Input: part model. Units: mm. Frame: model coordinates. Face numbers are marked on the shaded views. A direction names the side the tool comes from. Coordinates: 2 decimals unless noted, no trailing zeros. Write each loop counter-clockwise with the first axis right and the second up, starting at its lowest first coordinate (ties: lowest second). Pieces come first, ordered by that corner, then holes. Notation, with made-up numbers: (77.5, 45.5) - (94.5, 45.5) arc R28 ccw to (94.5, 81.5) - close; hole circle Ø2 at (61, 30). An arc over 180 degrees is marked (long way). Use a Markdown table: item, result. Add a question column.
Q1. Section query A-A (z = 35). Return the cut outline in (x, y).
Q2. Pin query (flat end, axial travel): P1, Ø1.5, axis at x = -2, y = -1, coming from the -Z side; P2, Ø1.6, axis at y = 1.5, z = -39.5, coming from the -X side; P3, Ø3, axis at y = -3.5, z = -8, coming from the -X side. Return the tip coordinate at first contact, or that it passes through.
Q3. Section query B-B (x = 14). Return the cut outline in (y, z).
Q4. Material intervals for probe 1 along X at (y, z) = (2.1, 0); probe 2 along Z at (x, y) = (-23, 0.8); probe 3 along Z at (x, y) = (-24, 1.5), sorted ascending. Write a range as from..to.
Q5. Section query C-C (z = 18.5). Return the cut outline in (x, y), then the cut area to 3 significant figures.
Q6. Set-up query: the marked faces 1, 2 and 3. Return all of +Z, -Z, +X, -X, +Y, -Y with unobstructed straight access to the full face (end or side cutting, diameter ignored); none if empty.
Q7. Section query D-D (z = -5.5). Return the cut outline in (x, y), then the cut area to 3 significant figures.
from build123d import *

# Parameters (mm, degrees)
A_BASE_T42_OUTLINE_R              = 2.2479
A_BASE_T42_OUTLINE_R_2            = 1
A_BASE_T42_DEPTH                  = 3
OUTER_RIM_CUT_DEPTH               = 68.299702823
SKETCH2_W                         = 20
SKETCH2_H                         = 3
FLANGES_DEPTH                     = 3
CONTOURING_R                      = 1
SKETCH3_W                         = 15
SKETCH3_H                         = 3
BASE_SUPPORTS_DEPTH               = 3
BASE_SUPPORTS_CHAMFER_SIZE        = 3
SKETCH4_W                         = 3
SKETCH4_H                         = 45
DYNAMIXEL_SIDE_SUPPORTS_DEPTH     = 6.85
SKETCH5_W                         = 12
SKETCH5_H                         = 3
DYNAMIXEL_SIDE_SUPPORT_ENDS_DEPTH = 9.85
SKETCH8_W                         = 9
SKETCH8_H                         = 45
DYNAMIXEL_OFFSET_DEPTH            = 1.25
DYNAMIXEL_CONTOURING_R            = 1


# Read off the part's stored shape, not the designer's step: a_base_t42
with BuildPart() as part:
    # a_base_t42 outline → a_base_t42 (new body)
    with BuildSketch(Plane(origin=(0, 0, 0), x_dir=(1, 0, 0), z_dir=(0, 1, 0))):
        with BuildLine():
            ThreePointArc((31.5, -42), (52.5, 0), (31.5, 42))
            Line((31.5, 42), (-31.5, 42))
            ThreePointArc((-31.5, 42), (-52.5, 0), (-31.5, -42))
            Line((-31.5, -42), (31.5, -42))
        make_face()
        with Locations((-23, -35)):
            Circle(A_BASE_T42_OUTLINE_R, mode=Mode.SUBTRACT)
        with Locations((23, -35)):
            Circle(A_BASE_T42_OUTLINE_R, mode=Mode.SUBTRACT)
        with Locations((-40.25, 0)):
            Circle(A_BASE_T42_OUTLINE_R_2, mode=Mode.SUBTRACT)
        with Locations((-23, 35)):
            Circle(A_BASE_T42_OUTLINE_R, mode=Mode.SUBTRACT)
        with Locations((40.25, 0)):
            Circle(A_BASE_T42_OUTLINE_R_2, mode=Mode.SUBTRACT)
        with Locations((23, 35)):
            Circle(A_BASE_T42_OUTLINE_R, mode=Mode.SUBTRACT)
    extrude(amount=A_BASE_T42_DEPTH)

    # Sketch1 → Outer Rim Cut (cut, through all)
    with BuildSketch(Plane.XZ):
        with BuildLine():
            Line((31.5, 42), (-31.5, 42))
            ThreePointArc((-31.5, 42), (-52.5, 0), (-31.5, -42))
            Line((-31.5, -42), (31.5, -42))
            ThreePointArc((31.5, -42), (52.5, 0), (31.5, 42))
        make_face()
        with BuildLine():
            Line((30.483602149, 39), (-30.483602149, 39))
            ThreePointArc((-30.483602149, 39), (-49.5, 0), (-30.483602149, -39))
            Line((-30.483602149, -39), (30.483602149, -39))
            ThreePointArc((30.483602149, -39), (49.5, 0), (30.483602149, 39))
        make_face(mode=Mode.SUBTRACT)
    extrude(amount=-OUTER_RIM_CUT_DEPTH, mode=Mode.SUBTRACT)

    # Sketch2 → Flanges (add)
    with BuildSketch(Plane.XZ):
        with Locations((0, -40.5)):
            Rectangle(SKETCH2_W, SKETCH2_H)
        with Locations((0, 40.5)):
            Rectangle(SKETCH2_W, SKETCH2_H)
    extrude(amount=-FLANGES_DEPTH)

    # Contouring
    contouring_edges = [part.edges().sort_by_distance(p)[0] for p in [
        (30.483602149, 1.5, -39),
        (-30.483602149, 1.5, -39),
        (10, 1.5, -42),
        (-10, 1.5, -42),
        (30.483602149, 1.5, 39),
        (-30.483602149, 1.5, 39),
        (10, 1.5, 42),
        (-10, 1.5, 42),
    ]]
    fillet(contouring_edges, radius=CONTOURING_R)

    # Sketch3 → Base Supports (add)
    with BuildSketch(Plane.XZ):
        with Locations((0, -27)):
            Rectangle(SKETCH3_W, SKETCH3_H)
        with Locations((0, 27)):
            Rectangle(SKETCH3_W, SKETCH3_H)
    extrude(amount=BASE_SUPPORTS_DEPTH)

    # Base Supports Chamfer
    base_supports_chamfer_edges = [part.edges().sort_by_distance(p)[0] for p in [
        (0, 0, 28.5),
        (0, 0, -28.5),
    ]]
    chamfer(base_supports_chamfer_edges, length=BASE_SUPPORTS_CHAMFER_SIZE - 0.0001)  # a hair under: the kernel refuses the full size

    # Sketch4 → Dynamixel Side Supports (add)
    with BuildSketch(Plane.XZ):
        with Locations((-32.5, 0)):
            Rectangle(SKETCH4_W, SKETCH4_H)
        with Locations((32.5, 0)):
            Rectangle(SKETCH4_W, SKETCH4_H)
    extrude(amount=DYNAMIXEL_SIDE_SUPPORTS_DEPTH)

    # Sketch5 → Dynamixel Side Support Ends (add)
    with BuildSketch(Plane.XZ):
        with Locations((-28, 24)):
            Rectangle(SKETCH5_W, SKETCH5_H)
        with Locations((28, -24)):
            Rectangle(SKETCH5_W, SKETCH5_H)
    extrude(amount=DYNAMIXEL_SIDE_SUPPORT_ENDS_DEPTH)

    # Sketch8 → Dynamixel Offset (add)
    with BuildSketch(Plane.XZ):
        with Locations((-26.5, 0)):
            Rectangle(SKETCH8_W, SKETCH8_H)
        with Locations((26.5, 0)):
            Rectangle(SKETCH8_W, SKETCH8_H)
    extrude(amount=DYNAMIXEL_OFFSET_DEPTH)

    # Dynamixel Contouring
    dynamixel_contouring_edges = [part.edges().sort_by_distance(p)[0] for p in [
        (-31, -4.05, -22.5),
        (31, -4.05, 22.5),
        (-34, -4.925, 25.5),
        (-22, -5.55, 22.5),
        (-28, -9.85, 22.5),
        (34, -4.925, -25.5),
        (22, -5.55, -22.5),
        (28, -9.85, -22.5),
        (-22, -0.625, -22.5),
        (22, -0.625, 22.5),
    ]]
    fillet(dynamixel_contouring_edges, radius=DYNAMIXEL_CONTOURING_R)


solid = part.part
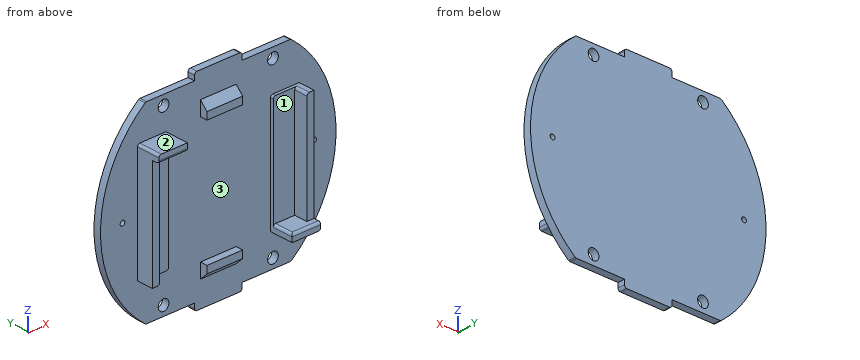
Values follow:
| question | item | result |
|---|---|---|
| 1 | outline | (-35, 0) - (-25.25, 0) - (-25.25, 3) - (-35, 3) - close; (-20.75, 0) - (20.75, 0) - (20.75, 3) - (-20.75, 3) - close; (25.25, 0) - (35, 0) - (35, 3) - (25.25, 3) - close |
| 2 | P1 | z = -31.25 |
| 2 | P2 | x = -30.86 |
| 2 | P3 | x = -34 |
| 3 | outline | (0, -39) - (3, -39) - (3, 39) - (0, 39) - close |
| 4 | probe 1 | -49.5..-41.25, -39.25..39.25, 41.25..49.5 |
| 4 | probe 2 | -39..-37.25, -32.75..32.75, 37.25..39 |
| 4 | probe 3 | -39..-37.01, -32.99..32.99, 37.01..39 |
| 5 | outline | (-45.91, 0) - (-34, 0) - (-34, -6.85) - (-31, -6.85) - (-31, -1.25) - (-22, -1.25) - (-22, 0) - (22, 0) - (22, -1.25) - (31, -1.25) - (31, -6.85) - (34, -6.85) - (34, 0) - (45.91, 0) - (45.91, 3) - (-45.91, 3) - close |
| 5 | area | 339 mm2 |
| 6 | face 1 | +Z, -Y |
| 6 | face 2 | +Z, -X, -Y |
| 6 | face 3 | -Y |
| 7 | outline | (-49.19, 0) - (-34, 0) - (-34, -6.85) - (-31, -6.85) - (-31, -1.25) - (-22, -1.25) - (-22, 0) - (22, 0) - (22, -1.25) - (31, -1.25) - (31, -6.85) - (34, -6.85) - (34, 0) - (49.19, 0) - (49.19, 3) - (-49.19, 3) - close |
| 7 | area | 359 mm2 |
